Work out the finished part from the listing and answer in its coordinate system (mm). Face numbers are marked on the shaded views. A direction names the side the tool comes from. Round coordinates to 2 decimals unless told otherwise and drop trailing zeros. Loops run counter-clockwise (first coordinate to the right, second up) from the corner with the lowest first, then second, coordinate; pieces in that order, holes last. Notation, with made-up numbers: (50.25, 12.5) - (81.25, 12.5) arc R17 ccw to (81.25, 26.5) - close; hole circle Ø6 at (11.25, -23.5). An arc over 180 degrees is marked (long way). Answer as CSV lines item,"result". Start each with the question number.
Q1. For the marked faces 1 and 2, determine the directions among +Z, -Z, +X, -X, +Y, -Y from which every point of the face is accessible in a straight line to the end or side of a thin tool.
Q2. Section B-B on z = -21.5 is taken. Write down the section's boundary in (x, y).
Q3. Each of these flat-tipped pins is pushed along its axis until it touches: pin 1 Ø10 at (x, y) = (24, -4.5) entering from +Z; pin 2 Ø5.5 at (x, z) = (94.5, -11.5) entering from +Y. Where does it stop, or does it pass through?
Q4. Straight lines are drawn through the part: L1, parallel to Z at x = 66.5, y = 0.5; L2, parallel to Y at x = 112.5, z = -8.25; L3, parallel to Y at x = 75.5, z = -18.75. For each, find the intervals that lie inside material, in ascending order. Write a range as [from, to].
Q5. Section A-A on x = 48.5 is taken. Write down the section's boundary in (y, z).
Q6. Section C-C on y = -12 is taken. Write down the section's boundary in (x, z).
Q7. Section D-D on x = 79.5 is taken. Write down the section's boundary in (y, z).
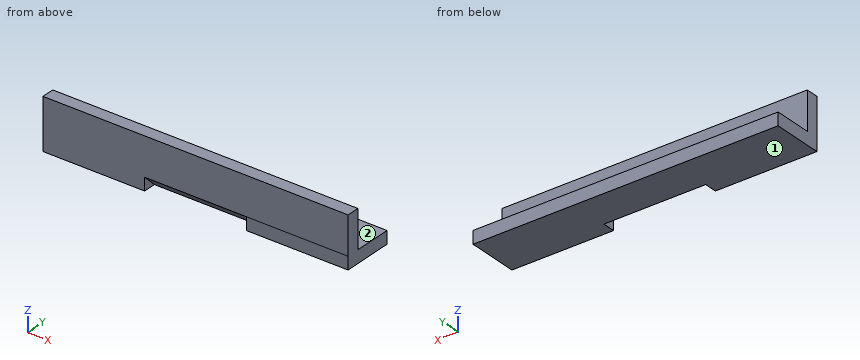
```python
from build123d import *

# Parameters (mm, degrees)
F1_DEPTH = 152.4
F3_DEPTH = 154.432
F5_DEPTH = 50.8
F7_DEPTH = 50.8


with BuildPart() as f1:
    # F0 (on Right) → F1 (new body)
    with BuildSketch(Plane.YZ):
        Polygon((-10.171386, 0.476147), (-16.521386, 0.476147), (-16.521386, -24.923853), (8.878614, -24.923853), (8.878614, -18.573853), (-10.171386, -18.573853), align=None)
    extrude(amount=F1_DEPTH)

    # F2 (on face) → F3 (cut)
    with BuildSketch(Plane(origin=(0, 0, 0), x_dir=(0, -1, 0), z_dir=(-1, 0, 0))):
        Polygon((10.171386, -24.923853), (16.521386, -24.923853), (16.521386, -18.573853), align=None)
    extrude(amount=-F3_DEPTH, mode=Mode.SUBTRACT)

    # F4 (on face) → F5 (join)
    with BuildSketch(Plane(origin=(0, 0, 0), x_dir=(0, -1, 0), z_dir=(-1, 0, 0))):
        Polygon((16.521386, -24.923853), (16.521386, -18.573853), (10.171386, -24.923853), align=None)
    extrude(amount=-F5_DEPTH)

    # F6 (on face) → F7 (join)
    with BuildSketch(Plane.YZ.offset(152.4)):
        Polygon((-16.522156, -24.923853), (-10.171386, -24.923853), (-16.521386, -18.573853), align=None)
    extrude(amount=-F7_DEPTH)


solid = f1.part
```
Findings:
1,face 1,"-Z, +X, -X, +Y, -Y"
1,face 2,"+Z, +X, -X, +Y"
2,outline,"(0, -16.52) - (50.8, -16.52) - (50.8, -13.6) - (101.6, -13.6) - (101.6, -16.52) - (152.4, -16.52) - (152.4, 8.88) - (0, 8.88) - close"
3,pin 1,"stops at z = -18.57"
3,pin 2,"stops at y = -10.17"
4,L1,"z = [-24.92, -18.57]"
4,L2,"y = [-16.52, -10.17]"
4,L3,"y = [-16.35, 8.88]"
5,outline,"(-16.52, -24.92) - (8.88, -24.92) - (8.88, -18.57) - (-10.17, -18.57) - (-10.17, 0.48) - (-16.52, 0.48) - close"
6,outline,"(0, -24.92) - (50.8, -24.92) - (50.8, -23.1) - (101.6, -23.1) - (101.6, -24.92) - (152.4, -24.92) - (152.4, 0.48) - (0, 0.48) - close"
7,outline,"(-16.52, -18.57) - (-10.17, -24.92) - (8.88, -24.92) - (8.88, -18.57) - (-10.17, -18.57) - (-10.17, 0.48) - (-16.52, 0.48) - close"
